from build123d import *

# Parameters (mm, degrees)
F1_DEPTH = 1
F2_SCALE = 3
F3_R     = 0.2


with BuildPart() as f1:
    # F0 (on Top) → F1 (new body)
    with BuildSketch(Plane.XY):
        with BuildLine():
            ThreePointArc((-0.5560147872, 0.5033364247), (0.1336825888, 0.7379898139), (0.6972442789, 0.2763157895))
            ThreePointArc((0.6972442789, 0.2763157895), (0.7707857892, 0.1845659616), (0.8831760866, 0.15))
            Line((0.8831760866, 0.15), (1.1, 0.15))
            ThreePointArc((1.1, 0.15), (1.25, 0), (1.1, -0.15))
            Line((1.1, -0.15), (0.8831760866, -0.15))
            ThreePointArc((0.8831760866, -0.15), (0.7707857892, -0.1845659616), (0.6972442789, -0.2763157895))
            ThreePointArc((0.6972442789, -0.2763157895), (0.1336825888, -0.7379898139), (-0.5560147872, -0.5033364247))
            ThreePointArc((-0.5560147872, -0.5033364247), (-0.6732626201, -0.4399801523), (-0.8042853971, -0.4643543905))
            Line((-0.8042853971, -0.4643543905), (-1.05, -0.6062177826))
            Line((-1.05, -0.6062177826), (-1, -0.692820323))
            Line((-1, -0.692820323), (-0.7542853971, -0.5509569309))
            ThreePointArc((-0.7542853971, -0.5509569309), (-0.6887740086, -0.5387698118), (-0.6301500921, -0.570447948))
            ThreePointArc((-0.6301500921, -0.570447948), (0.1515069339, -0.8363884558), (0.7902101828, -0.3131578947))
            ThreePointArc((0.7902101828, -0.3131578947), (0.8269809379, -0.2672829808), (0.8831760866, -0.25))
            Line((0.8831760866, -0.25), (1.1, -0.25))
            ThreePointArc((1.1, -0.25), (1.35, 0), (1.1, 0.25))
            Line((1.1, 0.25), (0.8831760866, 0.25))
            ThreePointArc((0.8831760866, 0.25), (0.8269809379, 0.2672829808), (0.7902101828, 0.3131578947))
            ThreePointArc((0.7902101828, 0.3131578947), (0.1515069339, 0.8363884558), (-0.6301500921, 0.570447948))
            ThreePointArc((-0.6301500921, 0.570447948), (-0.6887740086, 0.5387698118), (-0.7542853971, 0.5509569309))
            Line((-0.7542853971, 0.5509569309), (-1, 0.692820323))
            Line((-1, 0.692820323), (-1.05, 0.6062177826))
            Line((-1.05, 0.6062177826), (-0.8042853971, 0.4643543905))
            ThreePointArc((-0.8042853971, 0.4643543905), (-0.6732626201, 0.4399801523), (-0.5560147872, 0.5033364247))
        make_face()
        with BuildLine():
            Line((-0.949999984, 0.7794228911), (-1, 0.692820323))
            Line((-1, 0.692820323), (-0.7542853971, 0.5509569309))
            ThreePointArc((-0.7542853971, 0.5509569309), (-0.6887740086, 0.5387698118), (-0.6301500921, 0.570447948))
            ThreePointArc((-0.6301500921, 0.570447948), (0.1515069339, 0.8363884558), (0.7902101828, 0.3131578947))
            ThreePointArc((0.7902101828, 0.3131578947), (0.8269809379, 0.2672829808), (0.8831760866, 0.25))
            Line((0.8831760866, 0.25), (1.1, 0.25))
            ThreePointArc((1.1, 0.25), (1.35, 0), (1.1, -0.25))
            Line((1.1, -0.25), (0.8831760866, -0.25))
            ThreePointArc((0.8831760866, -0.25), (0.8269809379, -0.2672829808), (0.7902101828, -0.3131578947))
            ThreePointArc((0.7902101828, -0.3131578947), (0.1515069339, -0.8363884558), (-0.6301500921, -0.570447948))
            ThreePointArc((-0.6301500921, -0.570447948), (-0.6887740086, -0.5387698118), (-0.7542853971, -0.5509569309))
            Line((-0.7542853971, -0.5509569309), (-1, -0.692820323))
            Line((-1, -0.692820323), (-0.949999984, -0.7794228911))
            Line((-0.949999984, -0.7794228911), (-0.7042854035, -0.6375595118))
            ThreePointArc((-0.7042854035, -0.6375595118), (0.1693312868, -0.9347871287), (0.8831761083, -0.3500000319))
            Line((0.8831761083, -0.3500000319), (1.1, -0.3500000319))
            ThreePointArc((1.1, -0.3500000319), (1.4500000319, 0), (1.1, 0.3500000319))
            Line((1.1, 0.3500000319), (0.8831761083, 0.3500000319))
            ThreePointArc((0.8831761083, 0.3500000319), (0.1693312868, 0.9347871287), (-0.7042854035, 0.6375595118))
            Line((-0.7042854035, 0.6375595118), (-0.949999984, 0.7794228911))
        make_face()
    extrude(amount=F1_DEPTH)


with BuildPart() as f1_1:
    # F2: moved
    add(f1.part.scale(F2_SCALE))

    # F3
    f3_edges = [f1_1.edges().sort_by_distance(p)[0] for p in [
        (-2.112856, 1.912679, 1.5),
        (-2.112856, -1.912679, 1.5),
        (2.649528, -1.05, 1.5),
        (2.649528, 1.05, 1.5),
    ]]
    fillet(f3_edges, radius=F3_R)


solid = f1_1.part
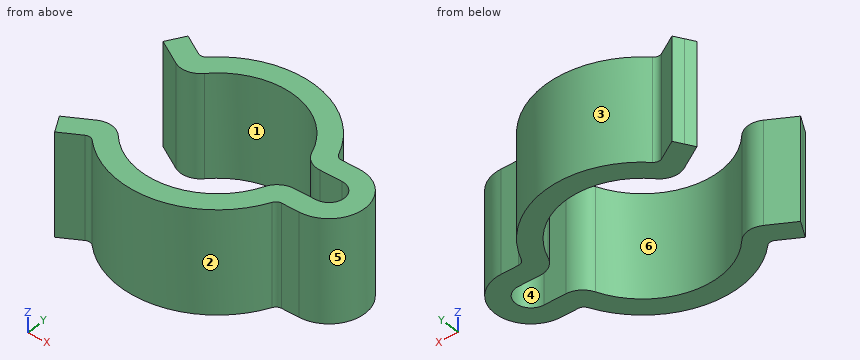
Verification items for the finished model (mm, model axes). Face numbers are marked on the shaded views. A direction names the side the tool comes from. Give positions to 0.01 mm unless a question says otherwise; leave off trailing zeros. Write each loop counter-clockwise with the first axis right and the second up, starting at its lowest first coordinate (ties: lowest second). Pieces come first, ordered by that corner, then holes.
(1) Cross-section at B-B (x = -2.5). Enter the section's corners in (y, z), plus the area to 3 significant figures.
(2) Cross-section at D-D (x = 0.25). Enter the section's corners in (y, z).
(3) Access from +Z, -Z, +X, -X, +Y, -Y to the whole of each face (thin tool, end or side, straight path). Record for the marked faces 5 and 6.
(4) Material ranges on line 1 (X direction, y = 2.05, z = 2.4); line 2 (Y direction, x = 3, z = 2.15); line 3 (X direction, y = 0, z = 0.8), recorded low to high.
(5) Cross-section at A-A (z = 2.1). Enter the section's corners in (x, y), plus the area to 3 significant figures.
(6) Gauge pin test, flat ends, axial feed: pin 1 (1 mm diameter, centred on y = -2, z = 0.5, fed in from +X); pin 2 (0.5 mm diameter, centred on x = 3, z = 2, fed in from -Y); pin 3 (3 mm diameter, centred on x = 2, y = 0, fed in from -Z); pin 4 (1.5 mm diameter, centred on x = 1, z = 2, fed in from +Y). Record the tip position at first contact, or that the pin passes through.
(7) Mould release check, pull along Y, two halves, no side actions. Record for the marked faces 1, 2, 3 and 4: +Y half, -Y half, draft (parallel to the pull), parting line (faces both ways), or undercut.
(8) Cross-section at C-C (y = 0). Enter the section's corners in (x, z).
Worked out:
1. outline: (-2.14, 0) - (-1.44, 0) - (-1.44, 3) - (-2.14, 3) - close; (1.44, 0) - (2.14, 0) - (2.14, 3) - (1.44, 3) - close
1. area: 4.16 mm2
2. outline: (-2.84, 0) - (-2.24, 0) - (-2.24, 3) - (-2.84, 3) - close; (2.24, 0) - (2.84, 0) - (2.84, 3) - (2.24, 3) - close
3. face 5: +Z, -Z, +X
3. face 6: +Z, -Z
4. line 1: x = -3.02 to -2.35, -1.98 to -0.93, 0.93 to 1.98
4. line 2: y = -1.05 to -0.45, 0.45 to 1.05
4. line 3: x = 3.75 to 4.35
5. outline: (-3.15, -1.82) - (-2.85, -2.34) - (-2.25, -1.99) arc R0.2 cw to (-2.01, -2.02) arc R2.85 ccw to (2.6, -1.17) arc R0.2 cw to (2.78, -1.05) - (3.3, -1.05) arc R1.05 ccw to (3.3, 1.05) - (2.78, 1.05) arc R0.2 cw to (2.6, 1.17) arc R2.85 ccw to (-2.01, 2.02) arc R0.2 cw to (-2.25, 1.99) - (-2.85, 2.34) - (-3.15, 1.82) - (-2.41, 1.39) arc R0.6 ccw to (-1.67, 1.51) arc R2.25 cw to (2.09, 0.83) arc R0.6 ccw to (2.65, 0.45) - (3.3, 0.45) arc R0.45 cw to (3.3, -0.45) - (2.65, -0.45) arc R0.6 ccw to (2.09, -0.83) arc R2.25 cw to (-1.67, -1.51) arc R0.6 ccw to (-2.41, -1.39) - close
5. area: 10.4 mm2
6. pin 1: stops at x = 2.42
6. pin 2: stops at y = -1.05
6. pin 3: stops at z = 0
6. pin 4: stops at y = 2.84
7. face 1: undercut
7. face 2: -Y half
7. face 3: +Y half
7. face 4: undercut
8. outline: (3.75, 0) - (4.35, 0) - (4.35, 3) - (3.75, 3) - close
